Autodesk Inventor part; units mm, degrees
ref_plane "YZ Plane" through (0, 0, 0) normal (1, 0, 0) x (0, 1, 0)
ref_plane "XZ Plane" through (0, 0, 0) normal (0, 1, 0) x (-1, 0, 0)
ref_plane "XY Plane" through (0, 0, 0) normal (0, 0, 1) x (1, 0, 0)
sketch "Esboço1" plane through (0, 0, 0) normal (0, 1, 0) x (-1, 0, 0)
  line L0 (20, -25) -> (-20, -25)
  line L1 (-20, -25) -> (-20, 25)
  line L2 (-20, 25) -> (20, 25)
  line L3 (20, 25) -> (20, -25)
  line L4 (20, -25) -> (-20, 25) construction
  line L5 (-20, -25) -> (20, 25) construction
  point P0 (0, 0)
  dimension "d0" = 40
  dimension "d1" = 50
extrude "Extrusão1" add sketch "Esboço1" along normal blind 40
chamfer "Chanfro1" distance 20 angle 30 1 edges at (0, 40, 25) measured on face at (-6.6667, 13.3333, 25)
chamfer "Chanfro2" distance 15 distance2 30 1 edges at (0, 40, -25) measured on face at (6.6667, 40, 0.6353)
properties part number "3D Model"
Model file for the job. Use its own axes, mm. Round coordinates to 2 decimals unless told otherwise and drop trailing zeros. Order: outer loops, then holes, each group sorted by start corner. A loop starts at its lowest first (then second) coordinate and runs counter-clockwise, first axis right, second up. Notation, with made-up numbers: M 14.25,51 L 73.25,51 A11 ccw 73.25,64 Z; hole C -12.5,29 d2. An arc over 180 degrees is marked long. Write each question's results on one line, items separated by ' | '. Start each with the question number.
(1) Saw through at B-B, the plane y = 14. Give the cut face in (x, z), then the cut area to 3 significant figures.
(2) Saw through at A-A, the plane x = -6.5. Give the cut face in (y, z), then the cut area to 3 significant figures.
(3) Probe probe 1 along Z at (x, y) = (-11, 33.5); probe 2 along Z at (x, y) = (13, 27.5); probe 3 along Y at (x, z) = (-12.5, 16.5). List the from-to ranges inside material, lowest first. Write a range as from..to.
(4) Saw through at C-C, the plane z = -21. Give the cut face in (x, y).
(5) Drop flat-ended pins along their axis: pin 1 (12 mm diameter, centred on x = 5.5, z = 19, fed in from +Y); pin 2 (1.5 mm diameter, centred on x = -4, y = 35.5, fed in from -Z) (3 decimals). Give the stop position or say it passes through.
Established:
1) outline: M -20,-23 L 20,-23 L 20,25 L -20,25 Z | area: 1,920 mm^2
2) outline: M 0,-25 L 10,-25 L 40,-10 L 40,13.45 L 20,25 L 0,25 Z | area: 1,660 mm^2
3) probe 1: z = -13.25..17.21 | probe 2: z = -16.25..20.67 | probe 3: y = 0..34.72
4) outline: M -20,0 L 20,0 L 20,18 L -20,18 Z
5) pin 1: stops at y = 40 | pin 2: stops at z = -12.625
